```python
from build123d import *

# Parameters (mm, degrees)
F0_W     = 20.66925
F0_H     = 7.60095
F1_DEPTH = 25.4


with BuildPart() as f1:
    # F0 (on Front) → F1 (new body)
    with BuildSketch(Plane.XZ):
        Polygon((-32.537401, 12.932173), (-60.807601, 11.065273), (-50.4063, -8.937228), (-32.537401, -14.804627), (17.0688, -14.804627), (48.5394, -14.804627), (48.5394, 4.397773), (48.5394, 9.198373), (27.87015, 9.198373), (7.2009, 9.198373), (0, 24.400273), (-11.2014, 24.400273), (-11.2014, 41.202374), (-14.4018, 41.202374), (-14.4018, 24.400273), (-32.537401, 24.400273), align=None)
        Polygon((-36.804602, 30.534372), (-32.537401, 24.400273), (-14.4018, 24.400273), align=None)
        Polygon((48.5394, 4.397773), (48.5394, -14.804627), (57.340499, -7.070328), (52.500348, -0.337245), (57.6072, 0), (55.206902, 4.397773), align=None)
        with Locations((17.535525, 12.998848)):
            Rectangle(F0_W, F0_H)
        Polygon((7.2009, 16.799323), (27.87015, 16.799323), (22.136101, 26.800573), (14.135102, 26.800573), align=None)
    extrude(amount=F1_DEPTH)


solid = f1.part
```
Here's how the part is built. I have some questions about the finished solid (model axes, mm). A direction names the side the tool comes from. Coordinates: 2 decimals unless noted, no trailing zeros. Order: outer loops, then holes, each group sorted by start corner. A loop starts at its lowest first (then second) coordinate and runs counter-clockwise, first axis right, second up. Notation, with made-up numbers: (8, 87.25) -> (65, 87.25) arc R18 cw to (65, 99.25) -> close; hole circle Ø2 at (78, -31.75). An arc over 180 degrees is marked (long way). Return JSON: item names as keys, results as strings.
1) Thinking about a two-plate mould opening in X: for faces 1 (the flat face through (10.717, -12.522, 21.87)), 2 (the flat face through (18, -13, 26.801)), 3 (the flat face through (-46.475, -12.522, 12.012)), which applies, +X half, -X half, draft (parallel to the pull), parting line (faces both ways), or undercut?
Conclusion:
{"face 1": "undercut", "face 2": "draft", "face 3": "-X half"}
2) If I drill on probe 1 along Z at (x, y) = (36, -1.5); probe 2 along X at (y, z) = (-20.75, 36); probe 3 along X at (y, z) = (-3.5, 18), over which ranges is the centre line in solid material (lowest first)?
Conclusion:
{"probe 1": "z = -14.8 to 9.2", "probe 2": "x = -14.4 to -11.2", "probe 3": "x = -32.54 to 3.03, 8.03 to 27.18"}
3) If we section it at B-B on y = -14.75: List the corners of the cut face in (x, z) for me, plus the area to 3 significant figures.
Conclusion:
{"outline": "(-60.81, 11.07) -> (-50.41, -8.94) -> (-32.54, -14.8) -> (48.54, -14.8) -> (57.34, -7.07) -> (52.5, -0.34) -> (57.61, 0) -> (55.21, 4.4) -> (48.54, 4.4) -> (48.54, 9.2) -> (27.87, 9.2) -> (27.87, 16.8) -> (22.14, 26.8) -> (14.14, 26.8) -> (7.2, 16.8) -> (7.2, 9.2) -> (0, 24.4) -> (-11.2, 24.4) -> (-11.2, 41.2) -> (-14.4, 41.2) -> (-14.4, 24.4) -> (-36.8, 30.53) -> (-32.54, 24.4) -> (-32.54, 12.93) -> close", "area": "3,560 mm²"}
4) If we section it at C-C on x = -2.5: List the corners of the cut face in (y, z) for me.
Conclusion:
{"outline": "(-25.4, -14.8) -> (0, -14.8) -> (0, 24.4) -> (-25.4, 24.4) -> close"}
5) If we section it at D-D on z = 28.5: List the corners of the cut face in (x, y) for me, plus the area to 3 significant figures.
Conclusion:
{"outline": "(-35.39, -25.4) -> (-29.37, -25.4) -> (-29.37, 0) -> (-35.39, 0) -> close; (-14.4, -25.4) -> (-11.2, -25.4) -> (-11.2, 0) -> (-14.4, 0) -> close", "area": "234 mm²"}
6) I'm going to push flat-ended pins straight in: P1, Ø5, axis at y = -19, z = 31, coming from the -X side; P2, Ø1.4, axis at y = -13.5, z = 6, coming from the +X side; P3, Ø8.5, axis at y = -13.5, z = 36, coming from the -X side. Where does each tip first touch, or does it pass through?
Conclusion:
{"P1": "stops at x = -36.8", "P2": "stops at x = 48.54", "P3": "stops at x = -14.4"}
7) On a 3-axis mill with a long thin cutter (end or side, diameter ignored), from which of +Z, -Z, +X, -X, +Y, -Y can I reach the whole of each face in a straight line? I mean faces 4 (the flat face through (-34.7, -12.52, 27.51)), 5 (the flat face through (48.539, -13, 7)), 6 (the flat face through (55.02, -12.52, -0.17)), 7 (the flat face through (-25.446, -12.522, 27.424)). Say none if no direction works.
Conclusion:
{"face 4": "-X, +Y, -Y", "face 5": "+Z, +X, +Y, -Y", "face 6": "+X, +Y, -Y", "face 7": "+Z, +Y, -Y"}
8) If we section it at A-A on z = 15: List the corners of the cut face in (x, y) for me, plus the area to 3 significant figures.
Conclusion:
{"outline": "(-32.54, -25.4) -> (4.45, -25.4) -> (4.45, 0) -> (-32.54, 0) -> close; (7.2, -25.4) -> (27.87, -25.4) -> (27.87, 0) -> (7.2, 0) -> close", "area": "1,460 mm²"}
